Verification items for the finished model (mm, model axes). A direction names the side the tool comes from. Coordinates: 2 decimals unless noted, no trailing zeros. Answer in a Markdown table with one row per item.
from build123d import *

# Parameters (mm, degrees)
F1_DEPTH = 7.62


with BuildPart() as f1:
    # F0 (on Front) → F1 (new body)
    with BuildSketch(Plane.XZ):
        with BuildLine():
            add(Edge.make_bspline(
                [(0, 0), (-3.4022271567, 9.5182356749), (-10.9690679678, 27.1009200022), (-28.1668864191, 25.8614681661), (-39.4263193011, 20.0893059373)],
                knots=[0, 0, 0, 0, 0.4995903231, 1, 1, 1, 1], degree=3))
            Line((0, 0), (0, 35.737555474))
            Line((0, 35.737555474), (-3.1367728952, 37.6913771033))
            Line((-3.1367728952, 37.6913771033), (-3.1367728952, 43.706933278))
            Line((-3.1367728952, 43.706933278), (-7.0221456699, 34.4971604645))
            Line((-7.0221456699, 34.4971604645), (-30.8036413044, 41.3585789502))
            Line((-30.8036413044, 41.3585789502), (-33.6170228571, 49.2606103394))
            add(Edge.make_bspline(
                [(-33.6170228571, 49.2606103394), (-41.4413912857, 49.3800380531), (-65.007380458, 36.5262842704), (-69.9772851484, 28.1731315931), (-78.3058434332, 16.9950854039)],
                knots=[0, 0, 0, 0, 0.5113918248, 1, 1, 1, 1], degree=3))
            add(Edge.make_bspline(
                [(-39.4263193011, 20.0893059373), (-40.7618194231, 23.0609141249), (-45.9085285726, 29.9278450611), (-60.4370668622, 31.9158113047), (-78.3058434332, 16.9950854039)],
                knots=[0, 0, 0, 0, 0.3412147066, 1, 1, 1, 1], degree=3))
        make_face()
        with BuildLine():
            Line((0, 35.737555474), (0, 0))
            add(Edge.make_bspline(
                [(0, 0), (3.4022271567, 9.5182356749), (10.9690679678, 27.1009200022), (28.1668864191, 25.8614681661), (39.4263193011, 20.0893059373)],
                knots=[0, 0, 0, 0, 0.4995903231, 1, 1, 1, 1], degree=3))
            add(Edge.make_bspline(
                [(39.4263193011, 20.0893059373), (40.7618194231, 23.0609141249), (45.9085285726, 29.9278450611), (60.4370668622, 31.9158113047), (78.3058434332, 16.9950854039)],
                knots=[0, 0, 0, 0, 0.3412147066, 1, 1, 1, 1], degree=3))
            add(Edge.make_bspline(
                [(33.6170228571, 49.2606103394), (41.4413912857, 49.3800380531), (65.007380458, 36.5262842704), (69.9772851484, 28.1731315931), (78.3058434332, 16.9950854039)],
                knots=[0, 0, 0, 0, 0.5113918248, 1, 1, 1, 1], degree=3))
            Line((33.6170228571, 49.2606103394), (30.8036413044, 41.3585789502))
            Line((30.8036413044, 41.3585789502), (7.0221456699, 34.4971604645))
            Line((7.0221456699, 34.4971604645), (3.1367728952, 43.706933278))
            Line((3.1367728952, 43.706933278), (3.1367728952, 37.6913771033))
            Line((3.1367728952, 37.6913771033), (0, 35.737555474))
        make_face()
    extrude(amount=F1_DEPTH)


solid = f1.part
1) Depth check by flat-ended pin: pin 1 (1 mm diameter, centred on x = 35.5, y = -3, fed in from -Z); pin 2 (3 mm diameter, centred on y = -6.5, z = 5.5, fed in from -X); pin 3 (3 mm diameter, centred on y = -3.5, z = 24.5, fed in from +X); pin 4 (1 mm diameter, centred on x = -44, z = 41.5, fed in from +Y). Enter the tip coordinate at first touch or a pass-through.
Response values:
| item | result |
|---|---|
| pin 1 | stops at z = 21.72 |
| pin 2 | stops at x = -2.68 |
| pin 3 | stops at x = 73.87 |
| pin 4 | stops at y = 0 |
2) Release check for a two-part mould opening along X. For faces 3 (the face through (3.137, -4, 41)), 4 (the face through (1, 0, 31)) record: +X half, -X half, draft (parallel to the pull), parting line (faces both ways), or undercut.
Response values:
| item | result |
|---|---|
| face 3 | undercut |
| face 4 | draft |
3) Tool access check on faces 1 (the face through (-3.137, -4, 41)), 2 (the face through (1, -7.62, 31)). Record the directions out of +Z, -Z, +X, -X, +Y, -Y that give a thin tool (end or side, any length) a straight path to the whole face; none if there is none.
Response values:
| item | result |
|---|---|
| face 1 | +Z, +Y, -Y |
| face 2 | +Z, -Z, +X, -X, -Y |
4) Thickness scan on L1, parallel to X at y = -2.5, z = 43; L2, parallel to X at y = -6.75, z = 2.5; L3, parallel to X at y = -6.5, z = 4.5. Record the ranges inside material, lowest first. Write a range as [from, to].
Response values:
| item | result |
|---|---|
| L1 | x = [-52.04, -31.39], [-3.44, -3.14], [3.14, 3.44], [31.39, 52.04] |
| L2 | x = [-0.91, 0.91] |
| L3 | x = [-1.67, 1.67] |
5) Sectioned sample at A-A (z = 26.5). Give the number of separate pieces and of enclosed holes in the cut face, then the cut area to 3 significant figures.
Response values:
| item | result |
|---|---|
| separate pieces | 3 |
| enclosed holes | 0 |
| area | 784 mm² |
